The listing builds one solid part. Answer for the finished solid, in the listing's coordinates (mm). A direction names the side the tool comes from. Give positions to 0.01 mm unless a question says otherwise; leave off trailing zeros. Write each loop counter-clockwise with the first axis right and the second up, starting at its lowest first coordinate (ties: lowest second). Pieces come first, ordered by that corner, then holes. Notation, with made-up numbers: (43, 50) - (83, 50) arc R11 cw to (83, 65) - close; hole circle Ø4 at (-26.75, 55). An arc over 180 degrees is marked (long way). Use a Markdown table: item, result. Add a question column.
from build123d import *

# Parameters (mm, degrees)
SKETCH_2_W           = 23.6
SKETCH_2_H           = 16
EXTRUDE_1_DEPTH      = 4
EXTRUDE_START        = 4
EXTRUDE_3_DEPTH      = 4.5
SKETCH_5_R           = 0.3
CUT_EXTRUDE_10_DEPTH = 1
EXTRUDE_2_DEPTH      = 2.5
SKETCH_6_W           = 4
SKETCH_6_H           = 2.95
CUT_EXTRUDE_11_DEPTH = 10
SKETCH_7_R           = 0.3
CUT_EXTRUDE_12_DEPTH = 24.50132975
SKETCH_8_W           = 13.6
SKETCH_8_H           = 2.95
CUT_EXTRUDE_13_DEPTH = 2.5
CUT_EXTRUDE_14_REACH = 25.022
SKETCH_9_R           = 0.3


with BuildPart() as part:
    # 草图2 → 凸台-拉伸1 (new body)
    with BuildSketch(Plane(origin=(0, 0, 0), x_dir=(0, 0, -1), z_dir=(1, 0, 0))):
        with Locations((5.8, 0)):
            Rectangle(SKETCH_2_W, SKETCH_2_H)
    extrude(amount=EXTRUDE_1_DEPTH)

    # 草图2<10> → 凸台-拉伸3 (add)
    with BuildSketch(Plane(origin=(0, 0, 0), x_dir=(0, 0, -1), z_dir=(1, 0, 0)).offset(EXTRUDE_START)):
        with BuildLine():
            ThreePointArc((0, -1.8), (1.272792206, -1.272792206), (1.8, 0))
            Line((1.8, 0), (0, 0))
            Line((0, 0), (0, -1.8))
        make_face()
        with BuildLine():
            Line((0, 0), (1.8, 0))
            ThreePointArc((1.8, 0), (1.272792206, 1.272792206), (0, 1.8))
            Line((0, 1.8), (0, 0))
        make_face()
        with BuildLine():
            Line((0, -1.8), (0, 0))
            Line((0, 0), (-1.8, 0))
            ThreePointArc((-1.8, 0), (-1.272792206, -1.272792206), (0, -1.8))
        make_face()
        with BuildLine():
            Line((-1.8, 0), (0, 0))
            Line((0, 0), (0, 1.8))
            ThreePointArc((0, 1.8), (-1.272792206, 1.272792206), (-1.8, 0))
        make_face()
    extrude(amount=EXTRUDE_3_DEPTH)

    # 草图5 → 切除-拉伸10 (cut)
    with BuildSketch(Plane(origin=(8.5, 0, 0), x_dir=(0, 0, -1), z_dir=(1, 0, 0))):
        Circle(SKETCH_5_R)
    extrude(amount=-CUT_EXTRUDE_10_DEPTH, mode=Mode.SUBTRACT)

    # 草图2<4> → 凸台-拉伸2 (add)
    with BuildSketch(Plane(origin=(0, 0, 0), x_dir=(0, 0, -1), z_dir=(1, 0, 0)).offset(EXTRUDE_START)):
        with BuildLine():
            ThreePointArc((-3.354101966, 3), (-1.837117307, 4.107919181), (0, 4.5))
            Line((0, 4.5), (-3.968626967, 4.5))
            ThreePointArc((-3.968626967, 4.5), (-4.643360347, 3.799895352), (-5.196152423, 3))
            Line((-5.196152423, 3), (-3.354101966, 3))
        make_face()
        with BuildLine():
            Line((0, 5), (1.8, 5))
            Line((1.8, 5), (1.8, 5.723635209))
            ThreePointArc((1.8, 5.723635209), (-1.245012655, 5.869407422), (-3.968626967, 4.5))
            Line((-3.968626967, 4.5), (0, 4.5))
            Line((0, 4.5), (0, 5))
        make_face()
        with BuildLine():
            ThreePointArc((0, 4.5), (0.919393397, 4.405078408), (1.8, 4.124318125))
            Line((1.8, 4.124318125), (1.8, 5))
            Line((1.8, 5), (0, 5))
            Line((0, 5), (0, 4.5))
        make_face()
        with BuildLine():
            ThreePointArc((1.8, 4.124318125), (3.764970119, 2.464751509), (4.5, 0))
            Line((4.5, 0), (6, 0))
            ThreePointArc((6, 0), (5.286764074, 2.837274331), (3.31662479, 5))
            Line((3.31662479, 5), (1.8, 5))
            Line((1.8, 5), (1.8, 4.124318125))
        make_face()
        with BuildLine():
            Line((1.8, 5.723635209), (1.8, 5))
            Line((1.8, 5), (3.31662479, 5))
            ThreePointArc((3.31662479, 5), (2.583771331, 5.415175501), (1.8, 5.723635209))
        make_face()
        with BuildLine():
            Line((6, 0), (4.5, 0))
            ThreePointArc((4.5, 0), (4.489038226, -0.313904132), (4.456206309, -0.626278954))
            Line((4.456206309, -0.626278954), (3.903880188, -4.556283516))
            ThreePointArc((3.903880188, -4.556283516), (5.262635021, -2.881782892), (5.941608412, -0.835038606))
            ThreePointArc((5.941608412, -0.835038606), (5.985384302, -0.418538842), (6, 0))
        make_face()
        with BuildLine():
            Line((5.356261262, -5), (5.941608412, -0.835038606))
            ThreePointArc((5.941608412, -0.835038606), (5.262635021, -2.881782892), (3.903880188, -4.556283516))
            Line((3.903880188, -4.556283516), (3.841519903, -5))
            Line((3.841519903, -5), (5.356261262, -5))
        make_face()
        Polygon((4.934638757, -8), (5.356261262, -5), (3.841519903, -5), (3.419897399, -8), align=None)
        with BuildLine():
            ThreePointArc((-5.196152423, 3), (-4.643360347, 3.799895352), (-3.968626967, 4.5))
            Line((-3.968626967, 4.5), (-6, 4.5))
            Line((-6, 4.5), (-6, 3))
            Line((-6, 3), (-5.196152423, 3))
        make_face()
    extrude(amount=EXTRUDE_2_DEPTH)

    # 草图6 → 切除-拉伸11 (cut)
    with BuildSketch(Plane(origin=(0, 0, -17.6), x_dir=(-1, 0, 0), z_dir=(0, 0, -1))):
        with Locations((-2, 6.525)):
            Rectangle(SKETCH_6_W, SKETCH_6_H)
        with Locations((-2, -6.525)):
            Rectangle(SKETCH_6_W, SKETCH_6_H)
    extrude(amount=-CUT_EXTRUDE_11_DEPTH, mode=Mode.SUBTRACT)

    # 草图7 → 切除-拉伸12 (cut, through all)
    with BuildSketch(Plane.XZ.offset(5.05)):
        with Locations((0, -9.6)):
            Circle(SKETCH_7_R)
        with Locations((0, -15.6)):
            Circle(SKETCH_7_R)
    extrude(amount=-CUT_EXTRUDE_12_DEPTH, mode=Mode.SUBTRACT)

    # 草图8 → 切除-拉伸13 (cut)
    with BuildSketch(Plane(origin=(6.5, 0, 0), x_dir=(0, 0, -1), z_dir=(1, 0, 0))):
        with Locations((0.8, -6.525)):
            Rectangle(SKETCH_8_W, SKETCH_8_H)
    extrude(amount=-CUT_EXTRUDE_13_DEPTH, mode=Mode.SUBTRACT)

    # 镜向1: part across plane


with BuildPart() as part_1:
    add(part.part)
    add(part.part.mirror(Plane(origin=(0, 0, 0), x_dir=(0, 0, 1), z_dir=(1, 0, 0))))

    # 草图9 → 切除-拉伸14 (cut, up to next)
    with BuildSketch(Plane.ZY.offset(4), mode=Mode.PRIVATE) as cut_extrude_14_sk1:
        with Locations((-14.1, -2)):
            Circle(SKETCH_9_R)
    cut_extrude_14_tool1 = extrude(cut_extrude_14_sk1.sketch, amount=-CUT_EXTRUDE_14_REACH, mode=Mode.PRIVATE) & part_1.part
    # 草图9 → 切除-拉伸14 (cut, up to next)
    with BuildSketch(Plane.ZY.offset(4), mode=Mode.PRIVATE) as cut_extrude_14_sk2:
        with Locations((-11.1, 2)):
            Circle(SKETCH_9_R)
    cut_extrude_14_tool2 = extrude(cut_extrude_14_sk2.sketch, amount=-CUT_EXTRUDE_14_REACH, mode=Mode.PRIVATE) & part_1.part
    add(cut_extrude_14_tool1.solids().sort_by_distance((-4, -2, -14.1))[0], mode=Mode.SUBTRACT)
    add(cut_extrude_14_tool2.solids().sort_by_distance((-4, 2, -11.1))[0], mode=Mode.SUBTRACT)


solid = part_1.part
1. The part is cut by section D-D (y = 1.25). Give the vertices of the cut face in (x, z), and give its area (3 significant figures).
2. Given P1, Ø0.6, axis at x = 4.5, z = 5.5, coming from the +Y side; P2, Ø6.5, axis at x = -2, z = -12.5, coming from the +Y side; P3, Ø1.7, axis at x = -5, z = -4.5, coming from the -Y side, each flat-ended and moving along its own axis, determine where each tip first touches the part or whether it passes through.
3. The part is cut by section C-C (x = -5.5). Give the vertices of the cut face in (y, z).
4. Which of the six approach directions +Z, -Z, +X, -X, +Y, -Y give full straight-line access (tool end or side, diameter ignored) to faces 1 (the flat face through (-5, -5.05, -5)), 2 (the flat face through (-5, 3, 5)), 3 (the flat face through (0, -5.05, -13)), 4 (the flat face through (5, -5.05, -5))?
5. The part is cut by section A-A (x = 2.5). Give the vertices of the cut face in (y, z), and give its area (3 significant figures).
6. The part is cut by section B-B (z = -11.1). Give the vertices of the cut face in (x, y), and give its area (3 significant figures).
7. Consider L1, parallel to Y at x = 1.5, z = -11.1; L2, parallel to X at y = -3.25, z = -3.75; L3, parallel to Y at x = 1.75, z = -12.25. Determine where each line is inside the solid, lowest interval first. Write a range as [from, to].
Check values:
| question | item | result |
|---|---|---|
| 1 | outline | (-8.5, -1.3) - (-4, -1.3) - (-4, -4.32) - (-6.5, -4.32) - (-6.5, -5.87) - (-4, -5.87) - (-4, -17.6) - (4, -17.6) - (4, -5.87) - (6.5, -5.87) - (6.5, -4.32) - (4, -4.32) - (4, -1.3) - (8.5, -1.3) - (8.5, 1.3) - (4, 1.3) - (4, 6) - (-4, 6) - (-4, 1.3) - (-8.5, 1.3) - close; hole circle Ø0.6 at (0, -15.6); hole circle Ø0.6 at (0, -9.6) |
| 1 | area | 219 mm2 |
| 2 | P1 | stops at y = 4.5 |
| 2 | P2 | stops at y = 5.05 |
| 2 | P3 | stops at y = -5.05 |
| 3 | outline | (-5.05, -5.35) - (-0.84, -5.94) arc R6 ccw to (4.5, 3.97) - (4.5, 6) - (3, 6) - (3, 3.35) arc R4.5 cw to (-0.63, -4.46) - (-5.05, -3.83) - close; circle Ø3.6 at (0, 0) |
| 4 | face 1 | +Z, -Z, -X, -Y |
| 4 | face 2 | +Z, -X, -Y |
| 4 | face 3 | -Z, +X, -X, -Y |
| 4 | face 4 | +Z, -Z, +X, -Y |
| 5 | outline | (-8, -7.6) - (-5.05, -7.6) - (-5.05, -17.6) - (5.05, -17.6) - (5.05, -7.6) - (8, -7.6) - (8, 6) - (-8, 6) - close; hole circle Ø0.6 at (-2, -14.1); hole circle Ø0.6 at (2, -11.1) |
| 5 | area | 318 mm2 |
| 6 | outline | (-4, -5.05) - (4, -5.05) - (4, 1.7) - (-4, 1.7) - close; (-4, 2.3) - (4, 2.3) - (4, 5.05) - (-4, 5.05) - close |
| 6 | area | 76.0 mm2 |
| 7 | L1 | y = [-5.05, 1.7], [2.3, 5.05] |
| 7 | L2 | x = [-4, 4] |
| 7 | L3 | y = [-5.05, 5.05] |
